Autodesk Inventor part; units mm, degrees
ref_plane "YZ Plane" through (0, 0, 0) normal (1, 0, 0) x (0, 1, 0)
ref_plane "XZ Plane" through (0, 0, 0) normal (0, 1, 0) x (-1, 0, 0)
ref_plane "XY Plane" through (0, 0, 0) normal (0, 0, 1) x (1, 0, 0)
sketch "Sketch1" plane through (0, 0, 0) normal (0, 1, 0) x (-1, 0, 0)
  line L0 (0, 15.85) -> (15, 15.85)
  line L1 (15, 15.85) -> (15, -15.85)
  line L2 (15, -15.85) -> (0, -15.85)
  line L3 (0, -15.85) -> (0, 15.85)
  point P0 (0, 0)
extrude "Extrusion1" add sketch "Sketch1" along normal blind 3
sketch "Sketch2" plane through (0, 3, 0) normal (0, 1, 0) x (1, 0, 0)
  line L0 (-15, 15.85) -> (-15, -15.85)
  line L1 (0, -15.85) -> (0, 15.85)
  line L2 (-15, -15.85) -> (0, -15.85)
  line L3 (0, -15.85) -> (0, -12.85)
  line L4 (0, -12.85) -> (-15, -12.85)
  line L5 (-15, -12.85) -> (-15, -15.85)
  line L6 (0, 15.85) -> (-15, 15.85)
  line L7 (0, 15.85) -> (-15, 15.85)
  line L8 (-15, 15.85) -> (-15, 12.85)
  line L9 (-15, 12.85) -> (0, 12.85)
  line L10 (0, 12.85) -> (0, 15.85)
  point P0 (0, 0)
  dimension "d5" = 3
  dimension "d6" = 3
extrude "Extrusion2" add sketch "Sketch2" along normal blind 35 contours L6 L1 L9 L0 | L4 L1 L2 L0
sketch "Sketch4" plane through (0, 0, -15.85) normal (0, 0, -1) x (-1, 0, 0)
  arc A0 (8.05, 6.1974) -> (6.95, 6.1974) centre (7.5, 7.15) ccw
  line L0 (8.05, 5) -> (12.75, 5)
  line L1 (2.25, 5) -> (6.95, 5)
  line L2 (1.4, 10.65) -> (1.4, 5.85)
  line L3 (6.95, 37.1) -> (2.25, 37.1)
  line L4 (12.75, 37.1) -> (8.05, 37.1)
  arc A1 (6.95, 35.9026) -> (8.05, 35.9026) centre (7.5, 34.95) ccw
  line L5 (6.95, 37.1) -> (6.95, 35.9026)
  line L6 (8.05, 35.9026) -> (8.05, 37.1)
  line L7 (13.6, 31.45) -> (13.6, 36.25)
  line L8 (13.6, 5.85) -> (13.6, 10.65)
  arc A2 (12.75, 5) -> (13.6, 5.85) centre (12.75, 5.85) ccw
  line L9 (8.05, 5) -> (8.05, 6.1974)
  line L10 (6.95, 6.1974) -> (6.95, 5)
  arc A3 (1.4, 5.85) -> (2.25, 5) centre (2.25, 5.85) ccw
  arc A4 (2.25, 37.1) -> (1.4, 36.25) centre (2.25, 36.25) ccw
  line L11 (1.4, 36.25) -> (1.4, 31.45)
  line L12 (1.4, 27.762) -> (1.4, 31.45)
  line L13 (1.4, 10.65) -> (1.4, 24.638)
  circle A5 centre (7.5, 26.2) radius 2.25
  line L14 (13.6, 31.45) -> (13.6, 27.762)
  line L15 (13.6, 24.638) -> (13.6, 10.65)
  line L16 (2.25, 9.8) -> (12.75, 9.8)
  line L17 (12.75, 32.3) -> (2.25, 32.3)
  arc A6 (2.25, 32.3) -> (1.4, 31.45) centre (2.25, 31.45) ccw
  arc A7 (13.6, 31.45) -> (12.75, 32.3) centre (12.75, 31.45) ccw
  arc A8 (13.6, 36.25) -> (12.75, 37.1) centre (12.75, 36.25) ccw
  arc A9 (1.4, 10.65) -> (2.25, 9.8) centre (2.25, 10.65) ccw
  arc A10 (12.75, 9.8) -> (13.6, 10.65) centre (12.75, 10.65) ccw
  line L18 (13.6, 24.638) -> (13.6, 27.762)
  line L19 (1.4, 27.762) -> (1.4, 24.638)
  line L20 (0, 3) -> (15, 3)
  line L21 (15, 3) -> (0, 3)
  line L22 (0, 3) -> (0, 5)
  line L23 (0, 0) -> (0, 38)
  line L24 (0, 5) -> (15, 5)
  line L25 (15, 5) -> (15, 3)
  line L26 (15, 0) -> (15, 38)
  line L27 (7.5, 5) -> (7.5, 3)
  line L28 (8.05, 5) -> (6.95, 5)
  line L29 (7.5, 5) -> (7.5, 4.3316)
  line L30 (12.75, 37.1) -> (13.6, 37.1)
  line L31 (13.6, 37.1) -> (13.6, 36.25)
  line L32 (13.6, 5.85) -> (13.6, 5)
  line L33 (1.4, 5.85) -> (1.4, 5)
  line L34 (1.4, 36.25) -> (1.4, 37.1)
  line L35 (1.4, 37.1) -> (2.25, 37.1)
  line L36 (2.25, 32.3) -> (1.4, 32.3)
  line L37 (12.75, 32.3) -> (13.6, 32.3)
  line L38 (13.6, 10.65) -> (13.6, 9.8)
  line L39 (13.6, 9.8) -> (12.75, 9.8)
  line L40 (1.4, 9.8) -> (2.25, 9.8)
  circle A11 centre (7.5, 34.95) radius 1.1
  circle A12 centre (7.5, 7.15) radius 1.1
  point P0 (6.95, 6.1974)
  point P1 (8.05, 6.1974)
  point P2 (8.05, 35.9026)
  point P3 (6.95, 35.9026)
  dimension "d9" = 2
extrude "Extrusion3" cut sketch "Sketch4" against normal up to surface (3 mm away) contours A12 A0 | L39 A10 L8 | A10 L16 A9 L13 L19 L12 A6 L17 A7 L14 L18 L15 | L2 A9 L40 | A7 L37 L7 | L11 L36 A6 | A1 A11 | A5
sketch "Sketch6" plane through (-15, 0, 15.85) normal (0, 0, 1) x (1, 0, 0)
  circle A0 centre (7.5, 15.9) radius 3
  line L0 (0, 0) -> (0, 38)
  line L1 (0, 0) -> (15, 0)
  line L2 (15, 0) -> (15, 38)
extrude "Extrusion5" add sketch "Sketch6" along normal blind 14
properties part number "head_p2"
Verification items for the finished model (mm, model axes). A direction names the side the tool comes from. Give positions to 0.01 mm unless a question says otherwise; leave off trailing zeros. Order: outer loops, then holes, each group sorted by start corner. A loop starts at its lowest first (then second) coordinate and runs counter-clockwise, first axis right, second up. Notation, with made-up numbers: (77, -2.75) - (107, -2.75) arc R23 ccw to (107, 20.25) - close; hole circle Ø2 at (19, 30.5). An arc over 180 degrees is marked (long way). Answer as CSV lines item,"result". Start each with the question number.
Item 1: Material ranges on L1, parallel to Y at x = -7.5, z = -14.35; L2, parallel to X at y = 34.95, z = -14.1; L3, parallel to Z at x = -11.75, y = 35.5, recorded low to high.
Item 2: Gauge pin test, flat ends, axial feed: pin 1 (1.8 mm diameter, centred on x = -7.5, y = 7.15, fed in from +Z); pin 2 (4.5 mm diameter, centred on x = -9, z = -2.5, fed in from +Y); pin 3 (1 mm diameter, centred on y = 30, z = 16.5, fed in from +X); pin 4 (4.5 mm diameter, centred on x = -9.5, y = 26, fed in from -Z). Record the tip position at first contact, or that the pin passes through.
Item 3: Access from +Z, -Z, +X, -X, +Y, -Y to the whole of each face (thin tool, end or side, straight path). Record for faces 5 (the face through (-5.89, 13.37, 22.75)), 6 (the face through (0, 15, -13)), 7 (the face through (-7, 3, 0)), 8 (the face through (-1.4, 21, -14)).
Item 4: Section check B-B, the plane x = -7.5. Record the boundary of the cut face in (y, z), plus the area to 3 significant figures.
Item 5: Section check A-A, the plane y = 20. Record the boundary of the cut face in (x, z).
Item 6: Section check C-C, the plane x = -13. Record the boundary of the cut face in (y, z).
Item 7: Mould release check, pull along Z, two halves, no side actions. Record for faces 1 (the face through (-7, 20, 12.85)), 2 (the face through (-7.49, 6.05, -14.37)), 3 (the face through (-1, 16, -12.85)), 4 (the face through (-8, 16, 29.85)): released by +Z, released by -Z, zero draft, split by the parting line, or undercut.
Item 8: Section check D-D, the plane y = 7.15. Record the boundary of the cut face in (x, z), plus the area to 3 significant figures.
Filled in:
1,L1,"0 to 6.05, 8.25 to 9.8, 32.3 to 33.85, 36.05 to 38"
1,L2,"-15 to -8.6, -6.4 to 0"
1,L3,"-15.85 to -12.85, 12.85 to 15.85"
2,pin 1,"z = 15.85"
2,pin 2,"y = 3"
2,pin 3,"through"
2,pin 4,"z = 12.85"
3,face 5,"+Z"
3,face 6,"+Z, -Z, +X, +Y, -Y"
3,face 7,"+X, -X, +Y"
3,face 8,"-Z"
4,outline,"(0, -15.85) - (6.05, -15.85) - (6.05, -12.85) - (3, -12.85) - (3, 12.85) - (38, 12.85) - (38, 15.85) - (18.9, 15.85) - (18.9, 29.85) - (12.9, 29.85) - (12.9, 15.85) - (0, 15.85) - close; (8.25, -15.85) - (9.8, -15.85) - (9.8, -12.85) - (8.25, -12.85) - close; (32.3, -15.85) - (33.85, -15.85) - (33.85, -12.85) - (32.3, -12.85) - close; (36.05, -15.85) - (38, -15.85) - (38, -12.85) - (36.05, -12.85) - close"
4,area,"308 mm^2"
5,outline,"(-15, -15.85) - (-13.6, -15.85) - (-13.6, -12.85) - (-15, -12.85) - close; (-15, 12.85) - (0, 12.85) - (0, 15.85) - (-15, 15.85) - close; (-1.4, -15.85) - (0, -15.85) - (0, -12.85) - (-1.4, -12.85) - close"
6,outline,"(0, -15.85) - (9.8, -15.85) - (9.8, -12.85) - (3, -12.85) - (3, 12.85) - (38, 12.85) - (38, 15.85) - (0, 15.85) - close; (32.3, -15.85) - (38, -15.85) - (38, -12.85) - (32.3, -12.85) - close"
7,face 1,"undercut"
7,face 2,"zero draft"
7,face 3,"undercut"
7,face 4,"released by +Z"
8,outline,"(-15, -15.85) - (-8.6, -15.85) - (-8.6, -12.85) - (-15, -12.85) - close; (-15, 12.85) - (0, 12.85) - (0, 15.85) - (-15, 15.85) - close; (-6.4, -15.85) - (0, -15.85) - (0, -12.85) - (-6.4, -12.85) - close"
8,area,"83.4 mm^2"
